Build history of the part. All positions in model axes, mm. A direction names the side the tool comes from. Give positions to 0.01 mm unless a question says otherwise; leave off trailing zeros. Loops run counter-clockwise (first coordinate to the right, second up) from the corner with the lowest first, then second, coordinate; pieces in that order, holes last. Notation, with made-up numbers: (50, -37.5) -> (61, -37.5) arc R10 ccw to (61, -28.5) -> close; hole circle Ø10 at (63.5, -38). An arc over 180 degrees is marked (long way). One line per question, with ' | ' between items. Start each with the question number.
(1) Mould opens along X. For faces 1 (the face through (-81.029, 53.396, 15.21)), 2 (the face through (-83, 56, 30)), 3 (the face through (-81.262, -54.272, 41.056)) say: pulls with the +X half, pulls with the -X half, needs draft (parallel to the pull), parting line crosses it, or undercut.
(2) 3-axis set-ups, long thin cutter, end or side, ignore diameter. For faces 4 (the face through (86, 3, 30)), 5 (the face through (0, 59, 30)), 6 (the face through (-83.849, -3.987, 37.605)), 7 (the face through (-0.656, 61.736, 41.056)): which of +Z, -Z, +X, -X, +Y, -Y reach the whole face in a straight line?
(3) Drill centre lines: L1, parallel to Y at x = -10, z = 16.5; L2, parallel to X at y = 18, z = 43.5; L3, parallel to X at y = 47, z = 9. Where is each one in solid material? Low to high. Write a range as from..to.
(4) Flat gauge pins, fed straight in: pin 1 Ø5 at (x, y) = (50.14, 12.95) entering from +Z; pin 2 Ø5 at (x, z) = (-25, 5) entering from -Y; pin 3 Ø3 at (y, z) = (-25.5, 7.5) entering from -X. Where does each tip first touch, or does it go through?
(5) Slice it at C-C, the plane y = -4.5. Write the cut outline in (x, z).
(6) Slice it at D-D, the plane x = 26.5. Write the cut outline in (y, z).
(7) Slice it at B-B, the plane x = 0. Write the cut outline in (y, z), then the cut area to 3 significant figures.
(8) Slice it at A-A, the plane z = 21.5. Write the cut outline in (x, y), then the cut area to 3 significant figures.
```python
from build123d import *

# Parameters (mm, degrees)
SKETCH1_W               = 165.1
SKETCH1_H               = 110
BOSS_EXTRUDE1_DEPTH     = 45
SHELL1_T                = -5
FILLET1_R               = 5.334
CUT_EXTRUDE1_DEPTH      = 1.2446
BOSS_EXTRUDE2_DEPTH     = 15
SKETCH4_R               = 3.025
CUT_EXTRUDE2_DEPTH      = 8
MIRROR3_COPY_1_DEPTH    = 15
MIRROR3_COPY_2_SKETCH_R = 3.025
MIRROR3_COPY_2_DEPTH    = 8
FILLET3_R               = 10
BOSS_EXTRUDE3_DEPTH     = 15
SKETCH6_R               = 3.025
CUT_EXTRUDE3_DEPTH      = 8
FILLET5_R               = 10
BOSS_EXTRUDE4_DEPTH     = 15
SKETCH8_R               = 3.025
CUT_EXTRUDE4_DEPTH      = 8
FILLET6_R               = 5
SKETCH9_R               = 5
SKETCH9_R_2             = 3.025
BOSS_EXTRUDE5_DEPTH     = 5


with BuildPart() as part:
    # Sketch1 → Boss-Extrude1 (new body)
    with BuildSketch(Plane.XY):
        Rectangle(SKETCH1_W, SKETCH1_H)
    extrude(amount=BOSS_EXTRUDE1_DEPTH)

    # Shell1
    shell1_openings = [part.faces().sort_by_distance(p)[0] for p in [
        (0, 0, 45),
    ]]
    offset(amount=SHELL1_T, openings=shell1_openings, kind=Kind.INTERSECTION)

    # Fillet1
    fillet1_edges = [part.edges().sort_by_distance(p)[0] for p in [
        (77.55, -50, 25),
        (77.55, 50, 25),
        (-77.55, 50, 25),
        (-77.55, -50, 25),
        (82.55, -55, 22.5),
        (-82.55, -55, 22.5),
        (-82.55, 55, 22.5),
        (82.55, 55, 22.5),
    ]]
    fillet(fillet1_edges, radius=FILLET1_R)

    # Sketch2 → Cut-Extrude1 (cut)
    with BuildSketch(Plane.XY.offset(45)):
        with BuildLine():
            Line((-77.216, -53.7827), (77.216, -53.7827))
            ThreePointArc((77.216, -53.7827), (80.126946486, -52.576946486), (81.3327, -49.666))
            Line((81.3327, -49.666), (81.3327, 49.666))
            ThreePointArc((81.3327, 49.666), (80.126946486, 52.576946486), (77.216, 53.7827))
            Line((77.216, 53.7827), (-77.216, 53.7827))
            ThreePointArc((-77.216, 53.7827), (-80.126946486, 52.576946486), (-81.3327, 49.666))
            Line((-81.3327, 49.666), (-81.3327, -49.666))
            ThreePointArc((-81.3327, -49.666), (-80.126946486, -52.576946486), (-77.216, -53.7827))
        make_face()
        with BuildLine():
            Line((-78.7673, 49.666), (-78.7673, -49.666))
            ThreePointArc((-78.7673, -49.666), (-78.31293475, -50.76293475), (-77.216, -51.2173))
            Line((-77.216, -51.2173), (77.216, -51.2173))
            ThreePointArc((77.216, -51.2173), (78.31293475, -50.76293475), (78.7673, -49.666))
            Line((78.7673, -49.666), (78.7673, 49.666))
            ThreePointArc((78.7673, 49.666), (78.31293475, 50.76293475), (77.216, 51.2173))
            Line((77.216, 51.2173), (-77.216, 51.2173))
            ThreePointArc((-77.216, 51.2173), (-78.31293475, 50.76293475), (-78.7673, 49.666))
        make_face(mode=Mode.SUBTRACT)
    extrude(amount=-CUT_EXTRUDE1_DEPTH, mode=Mode.SUBTRACT)

    # Sketch3 → Boss-Extrude2 (add)
    with BuildSketch(Plane.XY.offset(45)):
        with BuildLine():
            ThreePointArc((80.987707571, 53.437707571), (82.143973426, 51.707233428), (82.55, 49.666))
            Line((82.55, 49.666), (82.55, 47.221825407))
            Line((82.55, 47.221825407), (87.551567689, 52.223393096))
            ThreePointArc((87.551567689, 52.223393096), (87.551567689, 60.001567689), (79.773393096, 60.001567689))
            Line((79.773393096, 60.001567689), (74.771825407, 55))
            Line((74.771825407, 55), (77.216, 55))
            ThreePointArc((77.216, 55), (79.257233428, 54.593973426), (80.987707571, 53.437707571))
        make_face()
    boss_extrude2 = extrude(amount=-BOSS_EXTRUDE2_DEPTH)

    # Sketch4 → Cut-Extrude2 (cut)
    with BuildSketch(Plane.XY.offset(45)):
        with Locations((83.662480392, 56.112480392)):
            Circle(SKETCH4_R)
    cut_extrude2 = extrude(amount=-CUT_EXTRUDE2_DEPTH, mode=Mode.SUBTRACT)

    # Mirror2: Boss-Extrude2, Cut-Extrude2 across plane
    add(boss_extrude2.mirror(Plane.ZX))
    add(cut_extrude2.mirror(Plane.ZX), mode=Mode.SUBTRACT)

    # Mirror3: Boss-Extrude2, Cut-Extrude2 across plane
    add(boss_extrude2.mirror(Plane(origin=(0, 0, 0), x_dir=(0, 0, 1), z_dir=(1, 0, 0))))
    add(cut_extrude2.mirror(Plane(origin=(0, 0, 0), x_dir=(0, 0, 1), z_dir=(1, 0, 0))), mode=Mode.SUBTRACT)

    # Mirror3 copy 1 sketch → Mirror3 copy 1 (add)
    with BuildSketch(Plane(origin=(0, 0, 45), x_dir=(-1, 0, 0), z_dir=(0, 0, 1))):
        with BuildLine():
            ThreePointArc((80.987707571, 53.437707571), (82.143973426, 51.707233428), (82.55, 49.666))
            Line((82.55, 49.666), (82.55, 47.221825407))
            Line((82.55, 47.221825407), (87.551567689, 52.223393096))
            ThreePointArc((87.551567689, 52.223393096), (87.551567689, 60.001567689), (79.773393096, 60.001567689))
            Line((79.773393096, 60.001567689), (74.771825407, 55))
            Line((74.771825407, 55), (77.216, 55))
            ThreePointArc((77.216, 55), (79.257233428, 54.593973426), (80.987707571, 53.437707571))
        make_face()
    extrude(amount=-MIRROR3_COPY_1_DEPTH)

    # Mirror3 copy 2 sketch → Mirror3 copy 2 (cut)
    with BuildSketch(Plane(origin=(0, 0, 45), x_dir=(-1, 0, 0), z_dir=(0, 0, 1))):
        with Locations((83.662480392, 56.112480392)):
            Circle(MIRROR3_COPY_2_SKETCH_R)
    extrude(amount=-MIRROR3_COPY_2_DEPTH, mode=Mode.SUBTRACT)

    # Fillet3
    fillet3_edges = [part.edges().sort_by_distance(p)[0] for p in [
        (82.55, 47.221825407, 37.5),
        (74.771825407, 55, 37.5),
        (82.55, -47.221825407, 37.5),
        (74.771825407, -55, 37.5),
        (-82.55, -47.221825407, 37.5),
        (-74.771825407, -55, 37.5),
        (-82.55, 47.221825407, 37.5),
        (-74.771825407, 55, 37.5),
    ]]
    fillet(fillet3_edges, radius=FILLET3_R)

    # Sketch5 → Boss-Extrude3 (add)
    with BuildSketch(Plane.XY.offset(45)):
        with BuildLine():
            Line((0, -55), (-5.5, -55))
            Line((-5.5, -55), (-5.5, -58.7827))
            ThreePointArc((-5.5, -58.7827), (0, -64.2827), (5.5, -58.7827))
            Line((5.5, -58.7827), (5.5, -55))
            Line((5.5, -55), (0, -55))
        make_face()
    boss_extrude3 = extrude(amount=-BOSS_EXTRUDE3_DEPTH)

    # Sketch6 → Cut-Extrude3 (cut)
    with BuildSketch(Plane.XY.offset(45)):
        with Locations((0, -58.7827)):
            Circle(SKETCH6_R)
    cut_extrude3 = extrude(amount=-CUT_EXTRUDE3_DEPTH, mode=Mode.SUBTRACT)

    # Mirror10: Boss-Extrude3, Cut-Extrude3 across plane
    add(boss_extrude3.mirror(Plane.ZX))
    add(cut_extrude3.mirror(Plane.ZX), mode=Mode.SUBTRACT)

    # Fillet5
    # the kernel refuses this fillet: 10 mm, written as the material it adds along each edge
    with BuildSketch(Plane(origin=(5.5, 55, 45), x_dir=(1, 0, 0), z_dir=(0, 0, -1)), Plane(origin=(-5.5, -55, 45), x_dir=(-1, 0, 0), z_dir=(0, 0, -1))) as fillet5_piece_1:
        with BuildLine():
            CenterArc((8.698421768, -10), FILLET5_R, 90, 66.352028346)
            Line((-0.46185034, -5.98883871), (-1.377877551, -5.587722581))
            ThreePointArc((-1.377877551, -5.587722581), (-1, -3.7827), (-1, 0))
            Line((-1, 0), (0, 1))
            Line((0, 1), (8.698421768, 1))
            Line((8.698421768, 1), (8.698421768, 0))
        make_face()
    extrude(amount=15)
    with BuildSketch(Plane(origin=(-5.5, 55, 45), x_dir=(-1, 0, 0), z_dir=(0, 0, -1)), Plane(origin=(5.5, -55, 45), x_dir=(1, 0, 0), z_dir=(0, 0, -1))) as fillet5_piece_2:
        with BuildLine():
            CenterArc((8.698421768, 10), FILLET5_R, 203.647971654, 66.352028346)
            Line((-0.46185034, 5.98883871), (-1.377877551, 5.587722581))
            ThreePointArc((-1.377877551, 5.587722581), (-1, 3.7827), (-1, 0))
            Line((-1, 0), (0, -1))
            Line((0, -1), (8.698421768, -1))
            Line((8.698421768, -1), (8.698421768, 0))
        make_face()
    extrude(amount=15)

    # Sketch7 → Boss-Extrude4 (add)
    with BuildSketch(Plane.XY.offset(45)):
        with BuildLine():
            Line((-82.55, 3.079689783), (-82.55, 8.579689783))
            Line((-82.55, 8.579689783), (-86.3327, 8.579689783))
            ThreePointArc((-86.3327, 8.579689783), (-91.8327, 3.079689783), (-86.3327, -2.420310217))
            Line((-86.3327, -2.420310217), (-82.55, -2.420310217))
            Line((-82.55, -2.420310217), (-82.55, 3.079689783))
        make_face()
    boss_extrude4 = extrude(amount=-BOSS_EXTRUDE4_DEPTH)

    # Sketch8 → Cut-Extrude4 (cut)
    with BuildSketch(Plane.XY.offset(45)):
        with Locations((-86.3327, 3.079689783)):
            Circle(SKETCH8_R)
    cut_extrude4 = extrude(amount=-CUT_EXTRUDE4_DEPTH, mode=Mode.SUBTRACT)

    # Mirror11: Boss-Extrude4, Cut-Extrude4 across plane
    add(boss_extrude4.mirror(Plane(origin=(0, 0, 0), x_dir=(0, 0, 1), z_dir=(1, 0, 0))))
    add(cut_extrude4.mirror(Plane(origin=(0, 0, 0), x_dir=(0, 0, 1), z_dir=(1, 0, 0))), mode=Mode.SUBTRACT)

    # Fillet6
    # the kernel refuses this fillet: 5 mm, written as the material it adds along each edge
    with BuildSketch(Plane(origin=(82.55, 8.579689783, 45), x_dir=(0, 1, 0), z_dir=(0, 0, -1)), Plane(origin=(-82.55, -2.420310217, 45), x_dir=(0, -1, 0), z_dir=(0, 0, -1))) as fillet6_piece_1:
        with BuildLine():
            CenterArc((4.929198469, 5), FILLET6_R, 186.657461203, 83.342538797)
            Line((-0.037086516, 4.420333333), (-0.533715015, 4.362366667))
            ThreePointArc((-0.533715015, 4.362366667), (-0.5, 3.7827), (-0.5, 0))
            Line((-0.5, 0), (0, -0.5))
            Line((0, -0.5), (4.929198469, -0.5))
            Line((4.929198469, -0.5), (4.929198469, 0))
        make_face()
    extrude(amount=15)
    with BuildSketch(Plane(origin=(82.55, -2.420310217, 45), x_dir=(0, -1, 0), z_dir=(0, 0, -1)), Plane(origin=(-82.55, 8.579689783, 45), x_dir=(0, 1, 0), z_dir=(0, 0, -1))) as fillet6_piece_2:
        with BuildLine():
            CenterArc((4.929198469, -5), FILLET6_R, 90, 83.342538797)
            Line((-0.037086516, -4.420333333), (-0.533715015, -4.362366667))
            ThreePointArc((-0.533715015, -4.362366667), (-0.5, -3.7827), (-0.5, 0))
            Line((-0.5, 0), (0, 0.5))
            Line((0, 0.5), (4.929198469, 0.5))
            Line((4.929198469, 0.5), (4.929198469, 0))
        make_face()
    extrude(amount=15)

    # Sketch9 → Boss-Extrude5 (add)
    # profile 1 of 4: a face of its own
    with BuildSketch(Plane.XY.offset(5)):
        with Locations((-60.35343772, -42.926)):
            Circle(SKETCH9_R)
        with Locations((-60.35343772, -42.926)):
            Circle(SKETCH9_R_2, mode=Mode.SUBTRACT)
    # profile 2 of 4: a face of its own
    with BuildSketch(Plane.XY.offset(5)):
        with Locations((50.13656228, -42.926)):
            Circle(SKETCH9_R)
        with Locations((50.13656228, -42.926)):
            Circle(SKETCH9_R_2, mode=Mode.SUBTRACT)
    # profile 3 of 4: a face of its own
    with BuildSketch(Plane.XY.offset(5)):
        with Locations((50.13656228, 12.954)):
            Circle(SKETCH9_R)
        with Locations((50.13656228, 12.954)):
            Circle(SKETCH9_R_2, mode=Mode.SUBTRACT)
    # profile 4 of 4: a face of its own
    with BuildSketch(Plane.XY.offset(5)):
        with Locations((-60.35343772, 42.799)):
            Circle(SKETCH9_R)
        with Locations((-60.35343772, 42.799)):
            Circle(SKETCH9_R_2, mode=Mode.SUBTRACT)
    extrude(amount=BOSS_EXTRUDE5_DEPTH)


solid = part.part
```
Final values:
1) face 1: pulls with the -X half | face 2: needs draft | face 3: undercut
2) face 4: -Z, +X, +Y, -Y | face 5: -Z, +X, -X, +Y | face 6: +Z, -Z, -X | face 7: +Z
3) L1: -55..-50, 50..55 | L2: -82.55..-77.55, 77.55..82.55 | L3: -82.55..-77.01, -63.06..-57.64, 77.01..82.55
4) pin 1: z = 5 | pin 2: y = -55 | pin 3: x = -82.55
5) outline: (-83.44, 30) -> (-82.55, 30) -> (-82.55, 0) -> (82.55, 0) -> (82.55, 30) -> (83.44, 30) -> (83.44, 45) -> (81.33, 45) -> (81.33, 43.76) -> (78.77, 43.76) -> (78.77, 45) -> (77.55, 45) -> (77.55, 5) -> (-77.55, 5) -> (-77.55, 45) -> (-78.77, 45) -> (-78.77, 43.76) -> (-81.33, 43.76) -> (-81.33, 45) -> (-83.44, 45) -> close
6) outline: (-55, 0) -> (55, 0) -> (55, 45) -> (53.78, 45) -> (53.78, 43.76) -> (51.22, 43.76) -> (51.22, 45) -> (50, 45) -> (50, 5) -> (-50, 5) -> (-50, 45) -> (-51.22, 45) -> (-51.22, 43.76) -> (-53.78, 43.76) -> (-53.78, 45) -> (-55, 45) -> close
7) outline: (-64.28, 30) -> (-55, 30) -> (-55, 0) -> (55, 0) -> (55, 30) -> (64.28, 30) -> (64.28, 45) -> (61.81, 45) -> (61.81, 37) -> (55.76, 37) -> (55.76, 45) -> (53.78, 45) -> (53.78, 43.76) -> (51.22, 43.76) -> (51.22, 45) -> (50, 45) -> (50, 5) -> (-50, 5) -> (-50, 45) -> (-51.22, 45) -> (-51.22, 43.76) -> (-53.78, 43.76) -> (-53.78, 45) -> (-55.76, 45) -> (-55.76, 37) -> (-61.81, 37) -> (-61.81, 45) -> (-64.28, 45) -> close | area: 1,130 mm2
8) outline: (-82.55, -49.67) arc R5.33 ccw to (-77.22, -55) -> (77.22, -55) arc R5.33 ccw to (82.55, -49.67) -> (82.55, 49.67) arc R5.33 ccw to (77.22, 55) -> (-77.22, 55) arc R5.33 ccw to (-82.55, 49.67) -> close; hole (-77.55, -44.67) arc R5.33 ccw to (-72.22, -50) -> (72.22, -50) arc R5.33 ccw to (77.55, -44.67) -> (77.55, 44.67) arc R5.33 ccw to (72.22, 50) -> (-72.22, 50) arc R5.33 ccw to (-77.55, 44.67) -> close | area: 2,650 mm2
